from build123d import *

# Parameters (mm, degrees)
F0_R     = 11
F0_R_2   = 10.5
F0_R_3   = 10.05
F1_DEPTH = 5
F0_R_4   = 4.5
F6_DEPTH = 0.5
F0_R_5   = 3.5
F7_DEPTH = 1


# Not quite as in the source:
# - a fillet or chamfer that OpenCascade refuses, or shapes differently, is made with other operations: its cross-section is extruded or revolved along the edge and cut away or added


with BuildPart() as f1:
    # F0 (on Top) → F1 (new body)
    with BuildSketch(Plane.XY):
        Circle(F0_R)
        Circle(F0_R_2, mode=Mode.SUBTRACT)
        Circle(F0_R_2)
        Circle(F0_R_3, mode=Mode.SUBTRACT)
    extrude(amount=F1_DEPTH)

    # F5: chamfer of 1 on 1 edges, made by hand

    # F5_s1 → F5_t2 (revolve, cut)
    with BuildSketch(Plane.XZ):
        Polygon((11, 4), (10, 5), (11, 5), align=None)
    revolve(axis=Axis((0, 0, 5), (0, 0, 1)), mode=Mode.SUBTRACT)

    # F0 (on Top) → F6 (join)
    with BuildSketch(Plane.XY):
        Circle(F0_R_3)
        Circle(F0_R_4, mode=Mode.SUBTRACT)
    extrude(amount=F6_DEPTH)

    # F0 (on Top) → F7 (join)
    with BuildSketch(Plane.XY):
        Circle(F0_R_4)
        Circle(F0_R_5, mode=Mode.SUBTRACT)
    extrude(amount=F7_DEPTH)


solid = f1.part
Verification items for the finished model (mm, model axes). A direction names the side the tool comes from. Coordinates: 2 decimals unless noted, no trailing zeros. Loops run counter-clockwise (first coordinate to the right, second up) from the corner with the lowest first, then second, coordinate; pieces in that order, holes last. Notation, with made-up numbers: M 87.5,56.25 L 126.5,56.25 A20 cw 126.5,90.25 Z; hole C -30.5,-14 d8. An arc over 180 degrees is marked long. One line per item, written item: value.
1. Section check A-A on x = 0. Record the cut outline in (y, z).
Answers follow:
outline: M -11,0 L -3.5,0 L -3.5,1 L -4.5,1 L -4.5,0.5 L -10.05,0.5 L -10.05,4.95 L -11,4 Z; M 3.5,0 L 11,0 L 11,4 L 10.05,4.95 L 10.05,0.5 L 4.5,0.5 L 4.5,1 L 3.5,1 Z
2. Set-up check for faces 4 (the cylindrical face through (9.586, 3.019, 2.694)), 5 (the cylindrical face through (3.233, -1.341, 0.493)): record each of +Z, -Z, +X, -X, +Y, -Y from which the full face is reachable in a straight line by a thin tool's end or side.
Answers follow:
face 4: +Z
face 5: +Z, -Z
3. Gauge pin test, flat ends, axial feed: P1, Ø10, axis at x = 3, y = 2.5, coming from the +Z side; P2, Ø2, axis at x = -8.5, z = 2, coming from the -Y side; P3, Ø1.5, axis at x = -8, z = 2.5, coming from the -Y side. Record the tip position at first contact, or that the pin passes through.
Answers follow:
P1: z = 1
P2: y = -8.05
P3: y = -8.27
4. Material ranges on line 1 along Y through (x, z) = (0, 0.65); line 2 along Y through (x, z) = (0, 0.4); line 3 along Y through (x, z) = (0, 3.4), recorded low to high. Write a range as from..to.
Answers follow:
line 1: -11..-10.05, -4.5..-3.5, 3.5..4.5, 10.05..11
line 2: -11..-3.5, 3.5..11
line 3: -11..-10.05, 10.05..11
5. Mould release check, pull along X, two halves, no side actions. Record for faces 1 (the flat face through (0, -4, 1)), 2 (the cylindrical face through (-2.38, -10.74, 1.97)), 3 (the flat face through (-3, 3, 0)): pulls with the +X half, pulls with the -X half, needs draft (parallel to the pull), parting line crosses it, or undercut.
Answers follow:
face 1: undercut
face 2: parting line crosses it
face 3: needs draft
